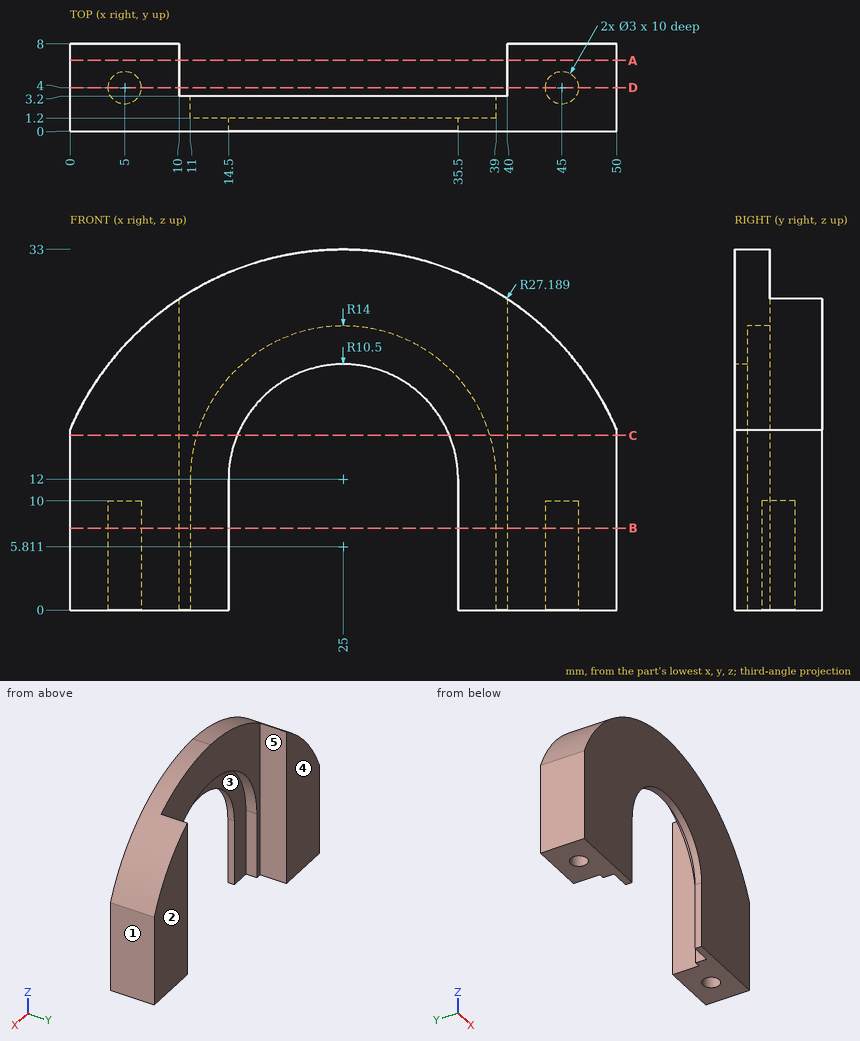
Here's the drawing with two shaded views (mm, measured from the low corner). I have some questions. A direction names the side the tool comes from. Round coordinates to 2 decimals unless told otherwise and drop trailing zeros. Write each loop counter-clockwise with the first axis right and the second up, starting at its lowest first coordinate (ties: lowest second). Pieces come first, ordered by that corner, then holes. Notation, with made-up numbers: M -25,63.5 L -16,63.5 A22 ccw -16,76.5 Z; hole C 28.25,57 d4. An arc over 180 degrees is marked long. Answer in a Markdown table with one row per item. Add a question column.
Q1. Will these pins go through, and if not, where does the flat tip stop? pin 1 Ø1.4 at (y, z) = (5.5, 15.5) entering from -X; pin 2 Ø1.5 at (x, y) = (20.5, 2.5) entering from -Z; pin 3 Ø15 at (x, z) = (20, 9) entering from +Y; pin 4 Ø4 at (y, z) = (5, 19) entering from +X.
Q2. On a 3-axis mill with a long thin cutter (end or side, diameter ignored), from which of +Z, -Z, +X, -X, +Y, -Y can I reach the whole of each face in a straight line? I mean the marked faces 4 and 5. Say none if no direction works.
Q3. If I drill on line 1 (Y direction, x = 5, z = 6); line 2 (X direction, y = 7, z = 12); line 3 (X direction, y = 2.75, z = 11), over which ranges is the centre line in solid material (lowest first)? Write a range as from..to.
Q4. If we mould it in two halves opening along X, with no side actions, what happens to the marked faces 1, 2 and 3? For each: +X half, -X half, draft (parallel to the pull), parting line (faces both ways), or undercut.
Q5. Imagine slicing it at D-D (y = 4). Please give me the cut outline in (x, z), then the cut area to 3 significant figures.
Q6. Imagine slicing it at C-C (z = 16). Please give me the cut outline in (x, y), then the cut area to 3 significant figures.
Q7. Imagine slicing it at A-A (y = 6.5). Please give me the cut outline in (x, z).
Q8. Imagine slicing it at B-B (z = 7.5). Please give me the cut outline in (x, y).
Values:
| question | item | result |
|---|---|---|
| 1 | pin 1 | x = 0 |
| 1 | pin 2 | z = 24.98 |
| 1 | pin 3 | y = 1.2 |
| 1 | pin 4 | x = 49.78 |
| 2 | face 4 | +Z, -Z, +X, -X, +Y |
| 2 | face 5 | +Z, -Z, +Y |
| 3 | line 1 | 0..2.5, 5.5..8 |
| 3 | line 2 | 0..10, 40..50 |
| 3 | line 3 | 0..11, 39..50 |
| 4 | face 1 | +X half |
| 4 | face 2 | draft |
| 4 | face 3 | undercut |
| 5 | outline | M 0,0 L 3.5,0 L 3.5,10 L 6.5,10 L 6.5,0 L 10,0 L 10,28.49 A27.19 ccw 0,16.5 Z; M 40,0 L 43.5,0 L 43.5,10 L 46.5,10 L 46.5,0 L 50,0 L 50,16.5 A27.19 ccw 40,28.49 Z |
| 5 | area | 414 mm^2 |
| 6 | outline | M 0,0 L 15.29,0 L 15.29,1.2 L 11.58,1.2 L 11.58,3.2 L 10,3.2 L 10,8 L 0,8 Z; M 34.71,0 L 50,0 L 50,8 L 40,8 L 40,3.2 L 38.42,3.2 L 38.42,1.2 L 34.71,1.2 Z |
| 6 | area | 179 mm^2 |
| 7 | outline | M 0,0 L 10,0 L 10,28.49 A27.19 ccw 0,16.5 Z; M 40,0 L 50,0 L 50,16.5 A27.19 ccw 40,28.49 Z |
| 8 | outline | M 0,0 L 14.5,0 L 14.5,1.2 L 11,1.2 L 11,3.2 L 10,3.2 L 10,8 L 0,8 Z; M 35.5,0 L 50,0 L 50,8 L 40,8 L 40,3.2 L 39,3.2 L 39,1.2 L 35.5,1.2 Z; hole C 5,4 d3; hole C 45,4 d3 |
